Source: CAD feature listing. Evaluate the final solid. Frame: model axes, mm. Face numbers are marked on the shaded views. A direction names the side the tool comes from. Give positions to 0.01 mm unless a question says otherwise; leave off trailing zeros. Order: outer loops, then holes, each group sorted by start corner. A loop starts at its lowest first (then second) coordinate and runs counter-clockwise, first axis right, second up.
Autodesk Inventor part; units mm, degrees
ref_plane "Work Plane1" through (29, 0, 0) normal (0, -1, 0) x (1, 0, 0)
ref_plane "YZ Plane" through (0, 0, 0) normal (1, 0, 0) x (0, 1, 0)
ref_plane "XZ Plane" through (0, 0, 0) normal (0, 1, 0) x (-1, 0, 0)
sketch "Skizze1" plane through (0, 0, 0) normal (0, 0, 1) x (1, 0, 0)
  line L0 (-2.6667, 0) -> (50, 0)
  line L1 (50, 0) -> (50, 6)
  line L2 (50, 6) -> (4.375, 6)
  line L3 (4.375, 6) -> (3.3014, 6)
  line L4 (3.3014, 6) -> (0, 6)
  line L5 (0, 6) -> (0, 9)
  line L6 (0, 9) -> (-12, 9)
  line L7 (-12, 9) -> (-12, 5.7735)
  line L8 (-12, 5.7735) -> (-6, 5.7735)
  line L9 (-6, 5.7735) -> (-2.6667, 0)
  line L10 (-24.4, 0) -> (62.4, 0)
  line L11 (0, -1.8) -> (0, 10.8)
  line L12 (4.375, 6) -> (0, 6) construction
  dimension "d1" = 45.625
  dimension "d2" = 1.0736
  dimension "d3" = 12
  dimension "d4" = 6
  dimension "d5" = 60
  dimension "d6" = 12
  dimension "d7" = 12
  dimension "d8" = 11.547
  dimension "d9" = 18
  dimension "d26" = 50
revolve "Körper" add sketch "Skizze1" angle 360 about axis through (-2.6667, 0, 0) along (1, 0, 0)
sketch "Skizze2" plane through (-12, 0, 0) normal (-1, 0, 0) x (0, 0, 1)
  circle A0 centre (0, 0) radius 5.7735
  line L0 (0, -12.6) -> (0, 12.6)
  line L1 (-12.6, 0) -> (12.6, 0)
  line L2 (5.7735, 0) -> (2.8868, -5)
  line L3 (2.8868, -5) -> (-2.8868, -5)
  line L4 (-2.8868, -5) -> (-5.7735, 0)
  line L5 (-5.7735, 0) -> (-2.8868, 5)
  line L6 (-2.8868, 5) -> (2.8868, 5)
  line L7 (2.8868, 5) -> (5.7735, 0)
extrude "Loch" add sketch "Skizze2" against normal up to next contours L7 A0 | A0 L2 | L6 L0 A0 | A0 L0 L3 | L0 L6 A0 | A0 L3 L0 | L4 A0 | A0 L5
fillet "Rundung1" radius 1.2 1 edges at (-12, -9, 0)
thread "Gewinde"
chamfer "Fase1" distance 1.0735 distance2 1.0735 1 edges at (50, -6, 0) measured on face at (50, 1.5551, -0.8476)
ref_plane "Work Plane1" through (29, 0, 0) normal (0, -1, 0) x (1, 0, 0)
fillet "Fillet2" radius 0.1 1 edges at (0, -6, 0)
equation "\"d1\" = GEL"
equation "\"d3\" = KOH"
equation "\"d4\" = INTI"
equation "\"d6\" = GD"
equation "\"d7\" = BDM"
equation "\"d8\" = 1.1547 * SW"
equation "\"d9\" = KOD"
equation "\"d26\" = NLG"
equation "\"d30\" = R"
equation "\"d17\" = RR"
equation "\"d13\" = GEL"
equation "\"d15\" = -0.5 * SPD + 0.5 * GD"
equation "\"d16\" = GUL"
equation "\"GD\" = 12"
equation "\"NLG\" = 50"
equation "\"GEL\" = 45.625"
equation "\"KOD\" = 18"
equation "\"KOH\" = 12"
equation "\"INTI\" = 6"
equation "\"GAL\" = 0.61345 * PTC"
equation "\"GUL\" = 0.61345 * PTC"
equation "\"BDM\" = NND"
equation "\"RR\" = 1.2"
equation "\"SPD\" = NND - 1.2269 * PTC"
equation "\"R\" = 0.1"
equation "\"TOA\" = 30deg"
equation "\"GD1\" = THREADDIA - 1.2269 * PTC"
equation "\"THREADDIA\" = 12"
equation "\"FAWI\" = 45deg"
equation "\"PTC\" = 1.75"
equation "\"NND\" = 12"
equation "\"E0\" = 1.155 * SW"
properties part number "ISO 4762 - M12 x 50" material "Edelstahl, 440C"
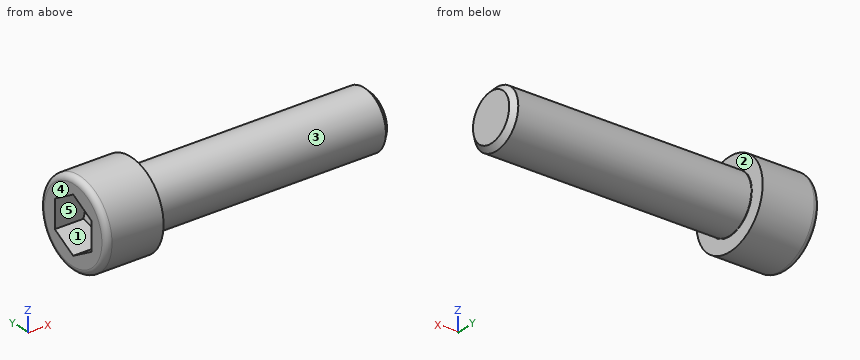
1) Material intervals for L1, parallel to Y at x = -8.5, z = 0.25; L2, parallel to X at y = 3, z = -7; L3, parallel to Y at x = -9, z = 5.5, sorted ascending.
Report:
L1: y = -9 to -5, 5 to 9
L2: x = -12 to 0
L3: y = -7.12 to -0.47, 0.47 to 7.12
2) Section query A-A, the plane x = -7. Return the cut outline in (y, z), and give its area (3 significant figures).
Report:
outline: circle Ø18 at (0, 0); hole (-5, -2.89) - (0, -5.77) - (5, -2.89) - (5, 2.89) - (0, 5.77) - (-5, 2.89) - close
area: 168 mm2
3) Pin query (flat end, axial travel): pin 1 (2 mm diameter, centred on x = 12.5, z = -6.5, fed in from -Y); pin 2 (1.5 mm diameter, centred on x = 23, y = -1, fed in from -Z); pin 3 (6 mm diameter, centred on x = 5, y = 4, fed in from +Z). Return the tip coordinate at first contact, or that it passes through.
Report:
pin 1: stops at y = -2.4
pin 2: stops at z = -5.99
pin 3: stops at z = 5.92
4) Section query B-B, the plane x = 46. Return the cut outline in (y, z), and give its area (3 significant figures).
Report:
outline: circle Ø12 at (0, 0)
area: 113 mm2
5) Reachability of the marked faces 4 and 5 from +Z, -Z, +X, -X, +Y, -Y: full face, straight path, thin tool, end or side. Return the list, or none.
Report:
face 4: +Z, -Z, -X, +Y, -Y
face 5: -X
6) Draft query along Z for the marked faces 1, 2 and 3. Return one class per face: +Z half, -Z half, draft (parallel to the pull), parting line (faces both ways), or undercut.
Report:
face 1: undercut
face 2: draft
face 3: parting line
